from build123d import *


with BuildPart() as f1:
    # F0 (on Front) → F1 (revolve)
    with BuildSketch(Plane.XZ):
        with BuildLine():
            Line((-4, 9.278649), (-2, 9.278649))
            Line((-2, 9.278649), (-2, 32.519547))
            Line((-2, 32.519547), (-3.7, 29.575061))
            Line((-3.7, 29.575061), (-3.2, 29.575061))
            Line((-3.2, 29.575061), (-3.2, 27.213341))
            Line((-3.2, 27.213341), (-3.7, 26.347315))
            Line((-3.7, 26.347315), (-3.2, 26.347315))
            Line((-3.2, 26.347315), (-3.2, 24.264861))
            Line((-3.2, 24.264861), (-3.7, 23.398835))
            Line((-3.7, 23.398835), (-3.2, 23.398835))
            Line((-3.2, 23.398835), (-3.2, 20.778649))
            ThreePointArc((-3.2, 20.778649), (-3.63934, 19.717989), (-4.7, 19.278649))
            Line((-4.7, 19.278649), (-5.25, 19.278649))
            Line((-5.25, 19.278649), (-4.5, 17.979611))
            Line((-4.5, 17.979611), (-4.5, 16.111982))
            Line((-4.5, 16.111982), (-5.25, 16.111982))
            Line((-5.25, 16.111982), (-4.5, 14.812944))
            Line((-4.5, 14.812944), (-4.5, 12.945316))
            Line((-4.5, 12.945316), (-5.25, 12.945316))
            Line((-5.25, 12.945316), (-4.5, 11.646278))
            Line((-4.5, 11.646278), (-4.5, 9.778649))
            ThreePointArc((-4.5, 9.778649), (-4.353553, 9.425096), (-4, 9.278649))
        make_face()
    revolve(axis=Axis((0, 0, 13.09317), (0, 0, 1)))


solid = f1.part
Input: part model. Units: mm. Frame: model coordinates. A direction names the side the tool comes from. Round coordinates to 2 decimals unless told otherwise and drop trailing zeros.
1) Contact query for flat-ended pins moving along their axis: P1, Ø3, axis at x = 4, z = 22.5, coming from the +Y side; P2, Ø6, axis at y = 3.5, z = 15.5, coming from the +X side; P3, Ø1.5, axis at y = -4, z = 17, coming from the -X side. Output: stop coordinate, or through.
2) Reachability of faces 4 (the cylindrical face through (2.539, 1.947, 25.292)), 5 (the flat face through (2, 1, 9.279)), 6 (the cylindrical face through (0.59, -4.46, 10.7)) from +Z, -Z, +X, -X, +Y, -Y: full face, straight path, thin tool, end or side. Return the list, or none.
3) Draft query along Y for faces 1 (the cylindrical face through (2.539, 1.947, 28.378)), 2 (the cylindrical face through (0, 2, 21)), 3 (the flat face through (-4, 3, 19.279)). Return one class per face: pulls with the +Y half, pulls with the -Y half, needs draft (parallel to the pull), parting line crosses it, or undercut.
4) Ray query, L1, parallel to Y at x = 0, z = 25.5; L2, parallel to Z at x = 1, y = 3.25. Return the intervals inside material, ascending.
Geometry says:
1. P1: stops at y = 2.42
1. P2: stops at x = 5.22
1. P3: stops at x = -3.11
2. face 4: none
2. face 5: -Z, +X, -X, +Y, -Y
2. face 6: -Z
3. face 1: parting line crosses it
3. face 2: undercut
3. face 3: needs draft
4. L1: y = -3.2 to -2, 2 to 3.2
4. L2: z = 9.28 to 20.03, 23.4 to 23.92, 26.35 to 26.87, 29.58 to 30.09
